```python
from build123d import *

# Parameters (mm, degrees)
SKETCH2_R           = 2.5
BOSS_EXTRUDE1_DEPTH = 2.5
CIRPATTERN1_COUNT   = 3


with BuildPart() as part:
    # Sketch1 → Revolve1 (revolve)
    with BuildSketch(Plane.XY):
        Polygon((-49.762825818, 0), (-49.762825818, 5), (-9.762825818, 5), (-5.567327662, 10), (2.732672338, 10), (0.206925517, 0), align=None)
    revolve(axis=Axis((-73.695652174, 0, 0), (1, 0, 0)))



with BuildPart() as body_2:
    # Sketch2 → Revolve2 (revolve)
    with BuildSketch(Plane.XY):
        with Locations((5.237174182, 31.25)):
            Circle(SKETCH2_R)
    revolve(axis=Axis((-155.619016335, 0, 0), (1, 0, 0)))


with BuildPart() as part_1:
    add(part.part)

    add(body_2.part)  # Boss-Extrude1 merges body 2
    # Sketch3 → Boss-Extrude1 (add, symmetric)
    with BuildSketch(Plane.XY):
        Polygon((1.837174182, 9.2), (-0.202790977, 9.2), (4.217209023, 31.2), (6.257174182, 31.2), align=None)
    boss_extrude1 = extrude(amount=BOSS_EXTRUDE1_DEPTH, both=True)

    # CirPattern1: Boss-Extrude1 ×3 about axis
    cirpattern1_axis = Axis((0, 0, 0), (1, 0, 0))
    for i in range(1, CIRPATTERN1_COUNT):
        add(boss_extrude1.rotate(cirpattern1_axis, i * 360 / CIRPATTERN1_COUNT))


solid = part_1.part
```
Build history of the part. All positions in model axes, mm. A direction names the side the tool comes from. Round coordinates to 2 decimals unless told otherwise and drop trailing zeros. Loops run counter-clockwise (first coordinate to the right, second up) from the corner with the lowest first, then second, coordinate; pieces in that order, holes last.
Item 1: Two-plate mould, pull along Y, no slides. Class faces 1 (the face through (-29.48, -1.08, -4.88)), 2 (the face through (-49.763, 0, 0)), 3 (the face through (3.882, 19.38, 0.035)): released by +Y, released by -Y, zero draft, split by the parting line, or undercut.
Item 2: Drill centre lines: line 1 along X through (y, z) = (9, -2); line 2 along X through (y, z) = (16.5, -1.5); line 3 along Z through (x, y) = (-14, -2.5). Where is each one in solid material? Low to high.
Item 3: Which spindle directions (+Z, -Z, +X, -X, +Y, -Y) get a long thin tool onto all of the face, cutting with end or side? Do faces 4 (the face through (3.885, -9.726, 16.776)), 5 (the face through (1.83, -9.69, 16.71)). Say none if no direction does.
Item 4: Pin check, flat tips, straight feed: P1, Ø4, axis at x = -12, z = 2, coming from the +Y side; P2, Ø4, axis at x = -1.5, y = 22, coming from the -Z side; P3, Ø6.5, axis at x = 4, y = 16, coming from the -Z side; P4, Ø1.8, axis at x = 4, y = 24, coming from the +Z side. Stop position of each tip, or through.
Item 5: Saw through at B-B (x = -12.5). List the corners of the cut face in (y, z).
Item 6: Saw through at A-A (y = 3). State how many separate pieces and enclosed holes the cut face has, then the cut area to 3 significant figures.
Worked answers:
1. face 1: split by the parting line
1. face 2: zero draft
1. face 3: undercut
2. line 1: x = -6.22 to 2.54
2. line 2: x = 1.26 to 3.3
2. line 3: z = -4.33 to 4.33
3. face 4: +X
3. face 5: -X
4. P1: stops at y = 5
4. P2: passes through
4. P3: stops at z = -31.17
4. P4: stops at z = 24.32
5. outline: circle Ø10 at (0, 0)
6. separate pieces: 3
6. enclosed holes: 0
6. area: 555 mm2
